```python
from build123d import *

# Parameters (mm, degrees)
F0_W      = 8
F0_H      = 8
F1_DEPTH  = 20
F3_DEPTH  = 15
F4_R      = 3.99999
F6_DEPTH  = 10
F7_R      = 3.125
F8_DEPTH  = 8.001
F9_DEPTH  = 25
F10_DEPTH = 27


# Not quite as in the source:
# - a fillet or chamfer is up to 0.001 mm smaller than in the source, because OpenCascade refuses the exact size


with BuildPart() as f1:
    # F0 (on Front) → F1 (new body)
    with BuildSketch(Plane.XZ):
        with Locations((4, 4)):
            Rectangle(F0_W, F0_H)
    extrude(amount=F1_DEPTH)

    # F2 (on face) → F3 (cut)
    with BuildSketch(Plane.XZ.offset(20)):
        Polygon((4.5, 8), (4, 8), (3.5, 8), (3.5, 0), (4.5, 0), align=None)
    extrude(amount=-F3_DEPTH, mode=Mode.SUBTRACT)

    # F4 (radius 4 in the source; OpenCascade refuses exactly that, so slightly less here)
    f4_edges = [f1.edges().sort_by_distance(p)[0] for p in [
        (1.75, -20, 8),
        (6.25, -20, 8),
        (6.25, -20, 0),
        (1.75, -20, 0),
        (8, 0, 4),
        (0, 0, 4),
    ]]
    fillet(f4_edges, radius=F4_R)

    # F5 (on face) → F6 (join)
    with BuildSketch(Plane.XY.offset(8)):
        with BuildLine():
            Line((3.5, -5), (3.5, -6.7041634566))
            ThreePointArc((3.5, -6.7041634566), (4, -6.75), (4.5, -6.7041634566))
            Line((4.5, -6.7041634566), (4.5, -5))
            Line((4.5, -5), (3.5, -5))
        make_face()
        with BuildLine():
            ThreePointArc((4.5, -6.7041634566), (6.1139418157, -5.7589059099), (6.75, -4))
            ThreePointArc((6.75, -4), (2.2410940901, -1.8860581843), (3.5, -6.7041634566))
            Line((3.5, -6.7041634566), (3.5, -5))
            Line((3.5, -5), (4.5, -5))
            Line((4.5, -5), (4.5, -6.7041634566))
        make_face()
    extrude(amount=-F6_DEPTH)

    # F7 (on face) → F8 (join, through all)
    with BuildSketch(Plane.YZ.offset(8)):
        with Locations((-16, 4)):
            Circle(F7_R)
    extrude(amount=-F8_DEPTH)

    # F9 (cut): a face of the model
    f9_faces = [f1.faces().sort_by_distance(p)[0] for p in [
        (4, -4, -2),
    ]]
    extrude(f9_faces, amount=-F9_DEPTH, mode=Mode.SUBTRACT)

    # F10 (cut): a face of the model
    f10_faces = [f1.faces().sort_by_distance(p)[0] for p in [
        (-0.001, -16, 4),
    ]]
    extrude(f10_faces, amount=-F10_DEPTH, mode=Mode.SUBTRACT)


solid = f1.part
```
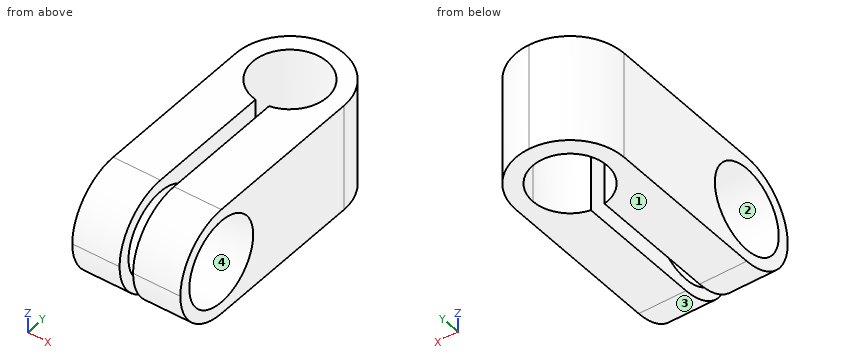
Verification items for the finished model (mm, model axes). Face numbers are marked on the shaded views. Coordinates: 2 decimals unless noted, no trailing zeros. Loops run counter-clockwise (first coordinate to the right, second up) from the corner with the lowest first, then second, coordinate; pieces in that order, holes last. Notation, with made-up numbers: (48, 2.5) -> (100, 2.5) arc R11 cw to (100, 16.5) -> close; hole circle Ø1 at (-35.5, -9). An arc over 180 degrees is marked (long way). Answer in a Markdown table with one row per item. Add a question column.
1. Depth check by flat-ended pin: P1, Ø1.5, axis at y = -15, z = 1.5, coming from the -X side. Enter the tip coordinate at first touch or a pass-through.
2. Material ranges on probe 1 along Z at (x, y) = (2.1, -16) (3 decimals); probe 2 along X at (y, z) = (-7.25, 5.5); probe 3 along X at (y, z) = (-4, 3), recorded low to high. Write a range as [from, to].
3. Section check A-A, the plane y = -9.25. Enter the section's corners in (x, z), then the cut area to 3 significant figures.
4. Draft check along Y on the marked faces 1, 2, 3 and 4. Enter one of: +Y half, -Y half, draft (parallel to the pull), parting line (faces both ways), or undercut.
5. Section check B-B, the plane x = 3. Give the number of separate pieces and of enclosed holes in the cut face, then the cut area to 3 significant figures.
Derived:
| question | item | result |
|---|---|---|
| 1 | P1 | stops at x = 0 |
| 2 | probe 1 | z = [0, 0.875], [7.125, 8] |
| 2 | probe 2 | x = [0, 3.5], [4.5, 8] |
| 2 | probe 3 | x = [0, 1.25], [6.75, 8] |
| 3 | outline | (0, 0) -> (3.5, 0) -> (3.5, 8) -> (0, 8) -> close; (4.5, 0) -> (8, 0) -> (8, 8) -> (4.5, 8) -> close |
| 3 | area | 56.0 mm² |
| 4 | face 1 | draft |
| 4 | face 2 | undercut |
| 4 | face 3 | -Y half |
| 4 | face 4 | undercut |
| 5 | separate pieces | 2 |
| 5 | enclosed holes | 1 |
| 5 | area | 80.4 mm² |
